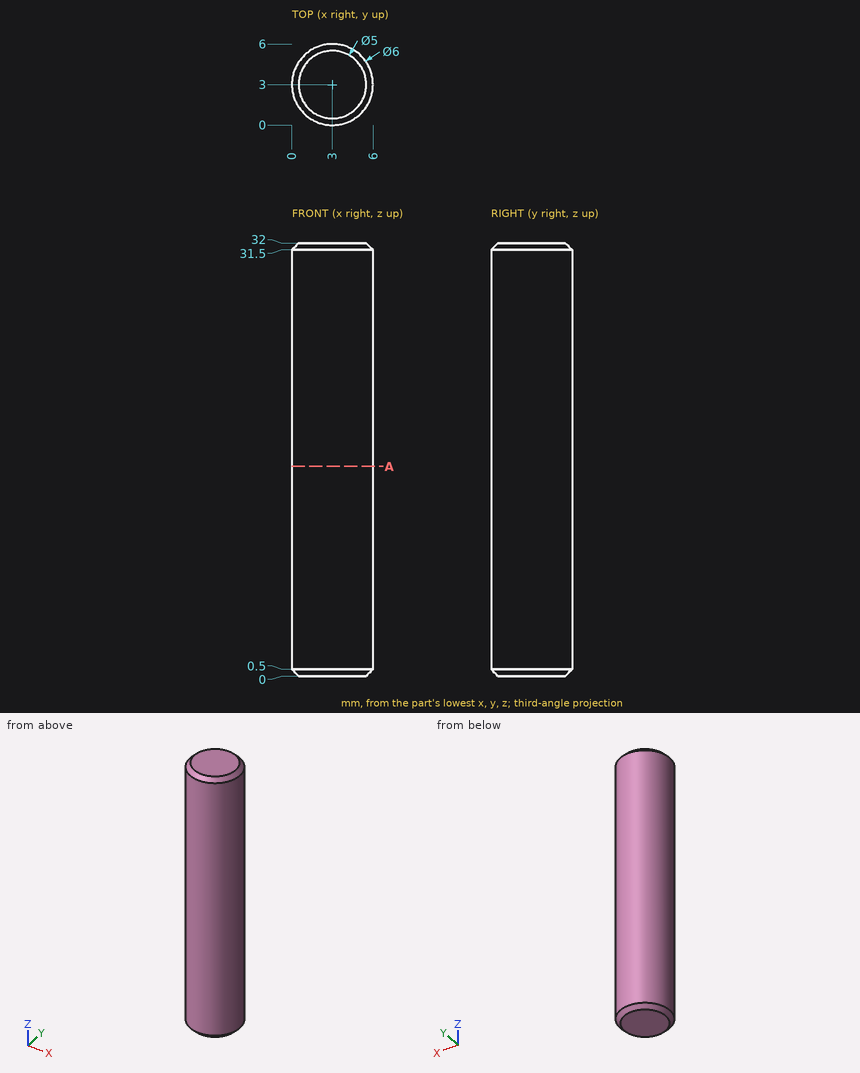
Study the drawing (mm; zero at the part's minimum x, y, z) and answer. Give positions to 0.01 mm unless a question says otherwise; leave off trailing zeros. Write each loop counter-clockwise with the first axis right and the second up, starting at its lowest first coordinate (ties: lowest second). Pieces come first, ordered by that corner, then holes. Notation, with made-up numbers: (40, 46) -> (55, 46) arc R11 ccw to (55, 52) -> close; hole circle Ø8 at (79.5, 83). An arc over 180 degrees is marked (long way). Write item = value, one per line. Start each with the question number.
1) Each of these flat-tipped pins is pushed along its axis until it touches: pin 1 (2 mm diameter, centred on x = 4.5, z = 4, fed in from -Y); pin 2 (1.5 mm diameter, centred on x = 5, z = 16, fed in from +Y). Where does it stop, or does it pass through?
2) The part is cut by section A-A, the plane z = 15.5. Determine the outline of the cut face in (x, y), and give its area (3 significant figures).
3) Straight lines are drawn through the part: line 1 along X through (y, z) = (3.2, 7.5); line 2 along X through (y, z) = (4.65, 6); line 3 along Y through (x, z) = (2.2, 15). For each, find the intervals that lie inside material, in ascending order.
Solutions:
q1.pin_1 = 0.04
q1.pin_2 = 5.73
q2.outline = circle Ø6 at (3, 3)
q2.area = 28.3 mm²
q3.line_1 = 0.01 to 5.99
q3.line_2 = 0.49 to 5.51
q3.line_3 = 0.11 to 5.89
